from build123d import *

# Parameters (mm, degrees)
SKETCH1_R           = 39.37
BOSS_EXTRUDE1_DEPTH = 3.175
SKETCH2_R           = 8.001
SKETCH2_R_2         = 1.8415
SKETCH2_R_3         = 2.5527
CUT_EXTRUDE1_DEPTH  = 4.175


with BuildPart() as part:
    # Sketch1 → Boss-Extrude1 (new body)
    with BuildSketch(Plane(origin=(0, 807.11642412, 0), x_dir=(-1, 0, 0), z_dir=(0, 1, 0))):
        Circle(SKETCH1_R)
    extrude(amount=-BOSS_EXTRUDE1_DEPTH)

    # Sketch2 → Cut-Extrude1 (cut, through all)
    with BuildSketch(Plane(origin=(0, 807.11642412, 0), x_dir=(1, 0, 0), z_dir=(0, 1, 0))):
        Circle(SKETCH2_R)
        with Locations((0, 11.176)):
            Circle(SKETCH2_R_2)
        with Locations((10.629007626, 3.453573929)):
            Circle(SKETCH2_R_2)
        with Locations((6.56908798, -9.041573929)):
            Circle(SKETCH2_R_2)
        with Locations((-6.56908798, -9.041573929)):
            Circle(SKETCH2_R_2)
        with Locations((-10.629007626, 3.453573929)):
            Circle(SKETCH2_R_2)
        with Locations((0, 28.702)):
            Circle(SKETCH2_R_3)
        with Locations((27.297224131, 8.869405773)):
            Circle(SKETCH2_R_3)
        with Locations((16.870612311, -23.220405773)):
            Circle(SKETCH2_R_3)
        with Locations((-16.870612311, -23.220405773)):
            Circle(SKETCH2_R_3)
        with Locations((-27.297224131, 8.869405773)):
            Circle(SKETCH2_R_3)
    extrude(amount=-CUT_EXTRUDE1_DEPTH, mode=Mode.SUBTRACT)


solid = part.part
Could you check a few things on this model? Use its own coordinates, in mm. Coordinates: 2 decimals unless noted, no trailing zeros. Write each loop counter-clockwise with the first axis right and the second up, starting at its lowest first coordinate (ties: lowest second). Pieces come first, ordered by that corner, then holes. Notation, with made-up numbers: M -26.5,2 L 14.5,2 A18 cw 14.5,8 Z; hole C 4.25,13 d8. An arc over 180 degrees is marked long. One line per question, with ' | ' between items.
1) Imagine slicing it at D-D, the plane y = 804.7. Give the number of separate pieces and of enclosed holes in the cut face, and give its area (3 significant figures).
Checks:
separate pieces: 1 | enclosed holes: 11 | area: 4,510 mm²
2) I need wall thicknesses on probe 1 along X at (y, z) = (805.7, 24); probe 2 along Z at (x, y) = (0, 804.95); probe 3 along Z at (x, y) = (5, 806.7). Which ranges of each line are inside material? Lowest first, please. Write a range as [from, to].
Checks:
probe 1: [-31.21, -19.3], [-14.44, 14.44], [19.3, 31.21] | probe 2: [-39.37, -31.25], [-26.15, -13.02], [-9.33, -8], [8, 39.37] | probe 3: [-39.05, -6.25], [6.25, 8.08], [10.01, 39.05]
3) Imagine slicing it at B-B, the plane x = 0. Write out the boundary of the cut face in (y, z), and give its area (3 significant figures).
Checks:
outline: M 803.94,-39.37 L 807.12,-39.37 L 807.12,-31.25 L 803.94,-31.25 Z; M 803.94,-26.15 L 807.12,-26.15 L 807.12,-13.02 L 803.94,-13.02 Z; M 803.94,-9.33 L 807.12,-9.33 L 807.12,-8 L 803.94,-8 Z; M 803.94,8 L 807.12,8 L 807.12,39.37 L 803.94,39.37 Z | area: 171 mm²
4) For pin 1 Ø2 at (x, z) = (10.63, -3.45) entering from -Y; pin 2 Ø1.5 at (y, z) = (805.5, 23.5) entering from -X; pin 3 Ø1 at (x, y) = (-5.5, 804.5) entering from +Z, each with a flat end and sliding along its axis, tell me the tip position at first contact or that it passes through.
Checks:
pin 1: through | pin 2: x = -32.13 | pin 3: z = 39.05
5) Imagine slicing it at C-C, the plane x = 28. Write out the boundary of the cut face in (y, z).
Checks:
outline: M 803.94,-27.68 L 807.12,-27.68 L 807.12,-11.32 L 803.94,-11.32 Z; M 803.94,-6.42 L 807.12,-6.42 L 807.12,27.68 L 803.94,27.68 Z
6) If we mould it in two halves opening along X, with no side actions, what happens to faces 1 (the face through (31.24, 805.55, -23.96)), 2 (the face through (-18.9, 805.55, 24.77)), 3 (the face through (0.6, 803.941, -8.2))? For each: released by +X, released by -X, zero draft, split by the parting line, or undercut.
Checks:
face 1: split by the parting line | face 2: undercut | face 3: zero draft
7) Imagine slicing it at A-A, the plane z = 0. Write out the boundary of the cut face in (x, y).
Checks:
outline: M -39.37,803.94 L -8,803.94 L -8,807.12 L -39.37,807.12 Z; M 8,803.94 L 39.37,803.94 L 39.37,807.12 L 8,807.12 Z
